```python
from build123d import *

# Parameters (mm, degrees)
BOSS_EXTRUDE2_DEPTH = 20


with BuildPart() as part:
    # Sketch1 → Revolve2 (revolve)
    with BuildSketch(Plane(origin=(0, 0, 0), x_dir=(0, 0, -1), z_dir=(1, 0, 0))):
        Polygon((-50, 0), (-50, 100), (0, 100), (0, 422.5), (-30, 422.5), (-30, 467.5), (-10, 467.5), (10.490381057, 462.009618943), (30, 442.5), (30, 0), align=None)
    revolve(axis=Axis((0, 0, -30), (0, 0, 1)))

    # Sketch2 → Boss-Extrude2 (add)
    with BuildSketch(Plane.XY):
        with BuildLine():
            ThreePointArc((20, 416.750824834), (21.571954346, 420.390674143), (25.299401198, 421.741852677))
            ThreePointArc((25.299401198, 421.741852677), (-14.324130925, 422.257112756), (-53.821656051, 419.057847248))
            ThreePointArc((-53.821656051, 419.057847248), (-30.183967117, 411.826133147), (-20, 389.302260461))
            Line((-20, 389.302260461), (-20, 101.980390272))
            ThreePointArc((-20, 101.980390272), (-21.066021038, 98.894323273), (-23.80952381, 97.124181211))
            ThreePointArc((-23.80952381, 97.124181211), (-7.6e-08, 100), (23.809523662, 97.124181247))
            ThreePointArc((23.809523662, 97.124181247), (21.066020991, 98.894323332), (20, 101.980390272))
            Line((20, 101.980390272), (20, 416.750824834))
        make_face()
        with BuildLine():
            Line((80.87262016, 65.265759081), (283.203155392, 306.393901336))
            ThreePointArc((283.203155392, 306.393901336), (286.746992321, 308.171754896), (290.470903088, 306.810861051))
            ThreePointArc((290.470903088, 306.810861051), (260.448719284, 332.675088673), (228.135411415, 355.612828872))
            ThreePointArc((228.135411415, 355.612828872), (241.594475451, 334.879000902), (234.917780585, 311.078585513))
            Line((234.917780585, 311.078585513), (50.230842435, 90.977263469))
            ThreePointArc((50.230842435, 90.977263469), (47.430537313, 89.298424107), (44.191066876, 89.705906207))
            ThreePointArc((44.191066876, 89.705906207), (64.278760914, 76.604444358), (80.669373607, 59.096972527))
            ThreePointArc((80.669373607, 59.096972527), (79.705554025, 62.216469562), (80.87262016, 65.265759081))
        make_face()
        with BuildLine():
            ThreePointArc((419.7278412, 48.319657717), (413.354719175, 87.430693327), (403.345384438, 125.772615671))
            ThreePointArc((403.345384438, 125.772615671), (400.328177931, 101.23826237), (379.914920814, 87.297783151))
            Line((379.914920814, 87.297783151), (96.958115442, 37.404863989))
            ThreePointArc((96.958115442, 37.404863989), (93.733820124, 37.918799861), (91.514166241, 40.313240718))
            ThreePointArc((91.514166241, 40.313240718), (97.855548193, 20.598341874), (100, 0))
            ThreePointArc((100, 0), (99.945767062, -3.292969231), (99.783127073, -6.582366715))
            ThreePointArc((99.783127073, -6.582366715), (101.049972403, -3.57316188), (103.904042548, -1.987446132))
            Line((103.904042548, -1.987446132), (413.892406924, 52.671866213))
            ThreePointArc((413.892406924, 52.671866213), (417.749925751, 51.755846586), (419.7278412, 48.319657717))
        make_face()
        with BuildLine():
            ThreePointArc((-252.561377668, 332.105405723), (-253.696840813, 335.904124837), (-251.709971685, 339.335144296))
            ThreePointArc((-251.709971685, 339.335144296), (-282.39456108, 314.260340916), (-310.59497249, 286.421041587))
            ThreePointArc((-310.59497249, 286.421041587), (-287.838996013, 296.075240754), (-265.55955831, 285.367081126))
            Line((-265.55955831, 285.367081126), (-80.87262016, 65.265759081))
            ThreePointArc((-80.87262016, 65.265759081), (-79.705554022, 62.216469491), (-80.669373691, 59.096972412))
            ThreePointArc((-80.669373691, 59.096972412), (-64.27876097, 76.604444311), (-44.191066878, 89.705906206))
            ThreePointArc((-44.191066878, 89.705906206), (-47.430537315, 89.298424108), (-50.230842435, 90.977263469))
            Line((-50.230842435, 90.977263469), (-252.561377668, 332.105405723))
        make_face()
        with BuildLine():
            ThreePointArc((-406.946479818, 92.064176334), (-410.25806463, 94.244302361), (-410.941451372, 98.149750609))
            ThreePointArc((-410.941451372, 98.149750609), (-418.329437639, 59.217662947), (-422.037449422, 19.764647353))
            ThreePointArc((-422.037449422, 19.764647353), (-410.8109597, 41.787452703), (-386.86084792, 47.90547303))
            Line((-386.86084792, 47.90547303), (-103.904042548, -1.987446132))
            ThreePointArc((-103.904042548, -1.987446132), (-101.049972452, -3.573161825), (-99.783127082, -6.582366568))
            ThreePointArc((-99.783127082, -6.582366568), (-98.480775309, 17.364817721), (-91.514166278, 40.313240634))
            ThreePointArc((-91.514166278, 40.313240634), (-93.733820164, 37.918799839), (-96.958115442, 37.404863989))
            Line((-96.958115442, 37.404863989), (-406.946479818, 92.064176334))
        make_face()
        with BuildLine():
            ThreePointArc((-370.916801355, -191.054904341), (-374.854980495, -191.513476599), (-377.888858856, -188.961002201))
            ThreePointArc((-377.888858856, -188.961002201), (-358.523321113, -223.533617647), (-336.003913346, -256.139845038))
            ThreePointArc((-336.003913346, -256.139845038), (-341.559909689, -232.053148883), (-327.14564731, -211.971638306))
            Line((-327.14564731, -211.971638306), (-78.317608663, -68.310703212))
            ThreePointArc((-78.317608663, -68.310703212), (-75.111985725, -67.690871012), (-72.207246346, -69.181743077))
            ThreePointArc((-72.207246346, -69.181743077), (-86.60254039, -49.999999979), (-96.016770169, -27.942438089))
            ThreePointArc((-96.016770169, -27.942438089), (-95.867649448, -28.63393708), (-95.817608663, -29.339560041))
            ThreePointArc((-95.817608663, -29.339560041), (-96.487481644, -31.839560041), (-98.317608663, -33.66968706))
            Line((-98.317608663, -33.66968706), (-370.916801355, -191.054904341))
        make_face()
        with BuildLine():
            ThreePointArc((-168.017869515, -387.654802013), (-130.960158095, -401.691034243), (-92.750411948, -412.193657258))
            ThreePointArc((-92.750411948, -412.193657258), (-112.489181919, -397.313503124), (-114.355362504, -372.664864277))
            Line((-114.355362504, -372.664864277), (-16.085495281, -102.67062307))
            ThreePointArc((-16.085495281, -102.67062307), (-14.028266101, -100.135269351), (-10.84479255, -99.41021313))
            ThreePointArc((-10.84479255, -99.41021313), (-34.202014712, -93.96926194), (-55.592060878, -83.123539189))
            ThreePointArc((-55.592060878, -83.123539189), (-53.961560514, -84.923661834), (-53.371663217, -87.27971662))
            ThreePointArc((-53.371663217, -87.27971662), (-53.447624452, -88.147957509), (-53.673200113, -88.989817337))
            Line((-53.673200113, -88.989817337), (-161.331029257, -384.777271937))
            ThreePointArc((-161.331029257, -384.777271937), (-164.053084938, -387.659971423), (-168.017869515, -387.654802013))
        make_face()
        with BuildLine():
            ThreePointArc((120.470548283, -404.96061166), (157.880718355, -391.892751619), (193.902038007, -375.377476225))
            ThreePointArc((193.902038007, -375.377476225), (169.21648425, -376.666453605), (151.943067336, -358.984058544))
            Line((151.943067336, -358.984058544), (53.673200113, -88.989817337))
            ThreePointArc((53.673200113, -88.989817337), (53.619435138, -85.725262282), (55.592060207, -83.123539638))
            ThreePointArc((55.592060207, -83.123539638), (34.202013938, -93.969262222), (10.844791714, -99.410213221))
            ThreePointArc((10.844791714, -99.410213221), (14.028265745, -100.135269129), (16.085495281, -102.67062307))
            Line((16.085495281, -102.67062307), (123.743324425, -398.45807767))
            ThreePointArc((123.743324425, -398.45807767), (123.511072308, -402.416057257), (120.470548283, -404.96061166))
        make_face()
        with BuildLine():
            ThreePointArc((352.589457658, -232.780850476), (372.847452038, -198.72349511), (389.825569397, -162.91800221))
            ThreePointArc((389.825569397, -162.91800221), (371.743876806, -179.772984263), (347.14564731, -177.330622155))
            Line((347.14564731, -177.330622155), (98.317608663, -33.66968706))
            ThreePointArc((98.317608663, -33.66968706), (96.178006763, -31.203452261), (96.016770156, -27.942438135))
            ThreePointArc((96.016770156, -27.942438135), (86.602540514, -49.999999765), (72.207246721, -69.181742686))
            ThreePointArc((72.207246721, -69.181742686), (75.111985993, -67.690870973), (78.317608663, -68.310703212))
            Line((78.317608663, -68.310703212), (350.916801355, -225.695920493))
            ThreePointArc((350.916801355, -225.695920493), (353.283026149, -228.877197545), (352.589457658, -232.780850476))
        make_face()
    extrude(amount=BOSS_EXTRUDE2_DEPTH)


solid = part.part
```
Here's how the part is built. I have some questions about the finished solid (model axes, mm). Give positions to 0.01 mm unless a question says otherwise; leave off trailing zeros. Loops run counter-clockwise (first coordinate to the right, second up) from the corner with the lowest first, then second, coordinate; pieces in that order, holes last. Notation, with made-up numbers: M 75.5,27 L 104.5,27 A33 cw 104.5,64 Z; hole C 89,-3.75 d2. An arc over 180 degrees is marked long. Put each result on its own line as item: value. Start each with the question number.
(1) Will these pins go through, and if not, where does the flat tip stop? pin 1 Ø10 at (y, z) = (256.5, 5.5) entering from -X; pin 2 Ø5 at (x, y) = (280.5, -329.5) entering from +Z; pin 3 Ø1.5 at (y, z) = (-367, 12) entering from -X.
(2) I need wall thicknesses on line 1 along X through (y, z) = (-4.5, 21); line 2 along X through (y, z) = (0, 21); line 3 along X through (y, z) = (110, 2.5). Which ranges of each line are inside material? Lowest first, please. Write a range as [from, to].
(3) If we mould it in two halves opening along Y, with no side actions, what happens to faces 1 (the flat face through (-6, -6, -30)), 2 (the cylindrical face through (-112.316, -397.625, 9.86)), 3 (the flat face through (-174.51, 176.86, 9.86))? For each: +Y half, -Y half, draft (parallel to the pull), parting line (faces both ways), or undercut.
(4) I want a section at A-A on x = 0. Please give me the cut outline in (y, z).
Answer block:
1. pin 1: x = -393.03
1. pin 2: z = 30
1. pin 3: x = -290.55
2. line 1: [-467.48, -422.48], [-99.9, 99.9], [422.48, 467.48]
2. line 2: [-467.5, -422.5], [-100, 100], [422.5, 467.5]
2. line 3: [-452.31, -407.93], [-118.41, -66.19], [-20, 20], [66.19, 118.41], [403.91, 452.31]
3. face 1: draft
3. face 2: undercut
3. face 3: undercut
4. outline: M -467.5,10 L -462.01,-10.49 L -442.5,-30 L 442.5,-30 L 462.01,-10.49 L 467.5,10 L 467.5,30 L 422.5,30 L 422.5,20 L 100,20 L 100,50 L -100,50 L -100,0 L -422.5,0 L -422.5,30 L -467.5,30 Z
